from build123d import *

# Parameters (mm, degrees)
EXTRUDE_1_DEPTH     = 40
SKETCH_2_R          = 1.85
CUT_EXTRUDE_1_DEPTH = 40
SKETCH_4_R          = 15.3
SKETCH_4_R_2        = 1.85
CUT_EXTRUDE_2_DEPTH = 40
FILLET_1_R          = 20


with BuildPart() as part:
    # ｽｹｯﾁ1 → ﾎﾞｽ - 押し出し1 (new body)
    with BuildSketch(Plane.XY):
        Polygon((0, 10), (0, 0), (60, 0), (60, -4), (-4, -4), (-4, 10), align=None)
    extrude(amount=EXTRUDE_1_DEPTH)

    # ｽｹｯﾁ2 → ｶｯﾄ - 押し出し1 (cut)
    with BuildSketch(Plane(origin=(0, 0, 0), x_dir=(0, 0, -1), z_dir=(1, 0, 0))):
        with Locations((-20, 5)):
            Circle(SKETCH_2_R)
    extrude(amount=-CUT_EXTRUDE_1_DEPTH, mode=Mode.SUBTRACT)

    # ｽｹｯﾁ4 → ｶｯﾄ - 押し出し2 (cut)
    with BuildSketch(Plane(origin=(0, 0, 0), x_dir=(1, 0, 0), z_dir=(0, 1, 0))):
        with Locations(Location((36, -20, 0), (0, 0, 270))):
            Circle(SKETCH_4_R)
        with Locations(Location((5, -5, 0), (0, 0, 270))):
            Circle(SKETCH_4_R_2)
        with Locations(Location((5, -35, 0), (0, 0, 270))):
            Circle(SKETCH_4_R_2)
    extrude(amount=-CUT_EXTRUDE_2_DEPTH, mode=Mode.SUBTRACT)

    # ﾌｨﾚｯﾄ1
    fillet_1_edges = [part.edges().sort_by_distance(p)[0] for p in [
        (60, -2, 0),
        (60, -2, 40),
    ]]
    fillet(fillet_1_edges, radius=FILLET_1_R - 0.0001)  # a hair under: the kernel refuses the full size


solid = part.part
Verification items for the finished model (mm, model axes). A direction names the side the tool comes from. Coordinates: 2 decimals unless noted, no trailing zeros. Loops run counter-clockwise (first coordinate to the right, second up) from the corner with the lowest first, then second, coordinate; pieces in that order, holes last. Notation, with made-up numbers: M 83,19.25 L 116,19.25 A29 cw 116,49.25 Z; hole C -18,2.5 d8. An arc over 180 degrees is marked long. One line per item, written item: value.
1. Mould release check, pull along Y, two halves, no side actions. Record for faces 1 (the flat face through (-4, 2.9, 19.7)), 2 (the flat face through (16, 0, 20)), 3 (the cylindrical face through (-1.97, 5.08, 21.85)): pulls with the +Y half, pulls with the -Y half, needs draft (parallel to the pull), parting line crosses it, or undercut.
Answers follow:
face 1: needs draft
face 2: pulls with the +Y half
face 3: undercut
2. Gauge pin test, flat ends, axial feed: P1, Ø2, axis at x = 5, z = 35, coming from the +Y side; P2, Ø5, axis at y = 4.5, z = 26.5, coming from the +X side; P3, Ø2, axis at x = 48.5, y = 0, coming from the +Z side; P4, Ø4, axis at x = 8.5, z = 8, coming from the +Y side. Record the tip position at first contact, or that the pin passes through.
Answers follow:
P1: through
P2: x = 0
P3: z = 38.54
P4: y = 0
3. Material ranges on line 1 along Y through (x, z) = (-1, 20); line 2 along X through (y, z) = (2.25, 36.5); line 3 along X through (y, z) = (-1.5, 17.5), recorded low to high. Write a range as from..to.
Answers follow:
line 1: -4..3.15, 6.85..10
line 2: -4..0
line 3: -4..20.91, 51.09..59.84
4. Section check A-A on x = 36. Record the cut outline in (y, z).
Answers follow:
outline: M -4,0 L 0,0 L 0,4.7 L -4,4.7 Z; M -4,35.3 L 0,35.3 L 0,40 L -4,40 Z
5. Section check C-C on x = 5. Record the cut outline in (y, z).
Answers follow:
outline: M -4,0 L 0,0 L 0,3.15 L -4,3.15 Z; M -4,6.85 L 0,6.85 L 0,33.15 L -4,33.15 Z; M -4,36.85 L 0,36.85 L 0,40 L -4,40 Z
6. Section check D-D on y = -2. Give the number of separate pieces and of enclosed holes in the cut face, plus the area to 3 significant figures.
Answers follow:
separate pieces: 1
enclosed holes: 3
area: 1,630 mm^2
7. Set-up check for faces 4 (the flat face through (0, 2.8, 19.7)), 5 (the flat face through (-2, 10, 20)): record each of +Z, -Z, +X, -X, +Y, -Y from which the full face is reachable in a straight line by a thin tool's end or side.
Answers follow:
face 4: +Z, -Z, +X, +Y
face 5: +Z, -Z, +X, -X, +Y
8. Section check B-B on y = 5. Record the cut outline in (x, z).
Answers follow:
outline: M -4,0 L 0,0 L 0,18.15 L -4,18.15 Z; M -4,21.85 L 0,21.85 L 0,40 L -4,40 Z
